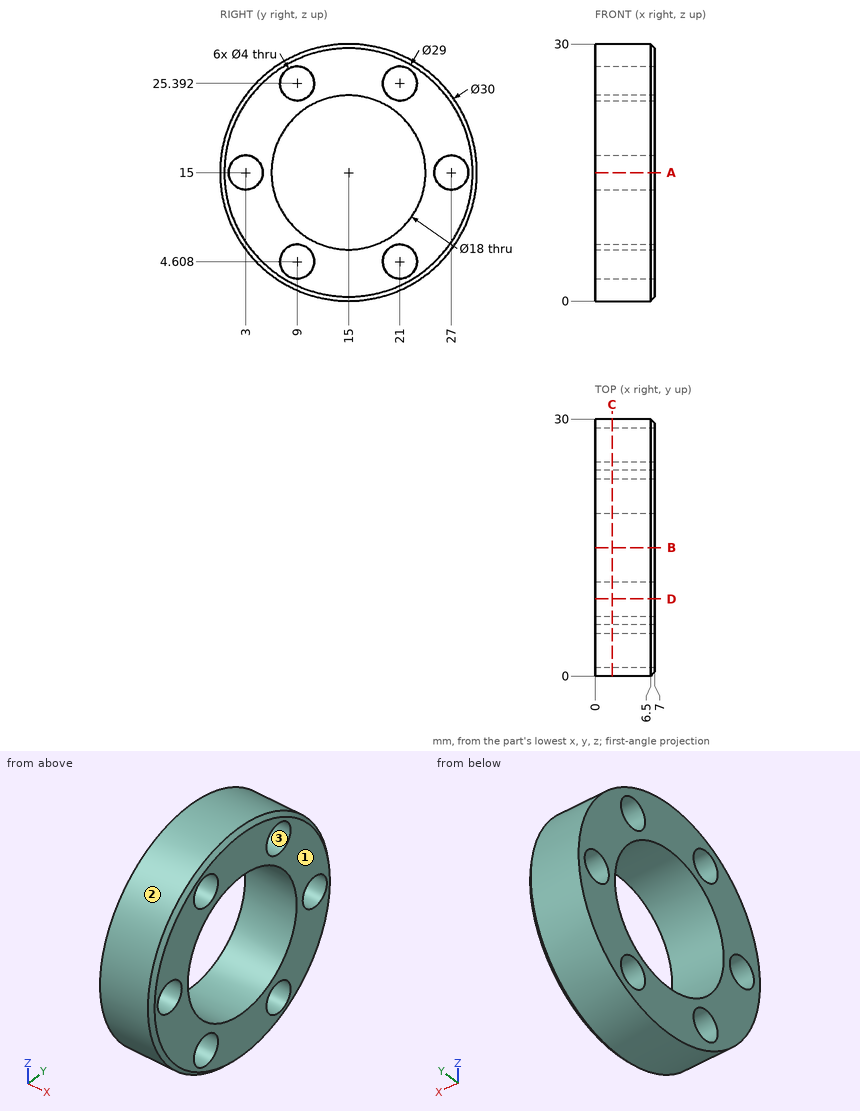
Check sheet for the drawn part. Datum: minimum x, y, z corner. Units: mm. Round coordinates to 2 decimals unless told otherwise and drop trailing zeros. Write each loop counter-clockwise with the first axis right and the second up, starting at its lowest first coordinate (ties: lowest second). Pieces come first, ordered by that corner, then holes. Notation, with made-up numbers: (73.25, -12) - (105.25, -12) arc R21 cw to (105.25, 8) - close; hole circle Ø1 at (59, 68.5). An arc over 180 degrees is marked (long way). Write each question's results on one line, items separated by ' | '.
(1) Depth check by flat-ended pin: pin 1 Ø2 at (x, z) = (4, 18.5) entering from -Y; pin 2 Ø1 at (x, z) = (1.5, 21) entering from -Y (1 decimal); pin 3 Ø2 at (x, z) = (6, 10.5) entering from +Y. Enter the tip coordinate at first touch or a pass-through.
Computed:
pin 1: stops at y = 0.21 | pin 2: stops at y = 1 | pin 3: stops at y = 29.59
(2) Thickness scan on probe 1 along Y at (x, z) = (3.5, 15); probe 2 along Z at (x, y) = (1, 22.5) (1 decimal); probe 3 along Y at (x, z) = (4.75, 5.25) (1 decimal). Record the ranges inside material, lowest first. Write a range as from..to.
Computed:
probe 1: y = 0..1, 5..6, 24..25, 29..30 | probe 2: z = 2..3.3, 5.9..10, 20..24.1, 26.7..28 | probe 3: y = 3.6..7.1, 10.9..19.1, 22.9..26.4
(3) Sectioned sample at D-D, the plane y = 9. Count the separate pieces of the cut face and the enclosed holes in it.
Computed:
separate pieces: 4 | enclosed holes: 0
(4) Draft check along Y on the marked faces 1, 2 and 3. Enter one of: pulls with the +Y half, pulls with the -Y half, needs draft (parallel to the pull), parting line crosses it, or undercut.
Computed:
face 1: needs draft | face 2: parting line crosses it | face 3: undercut
(5) Sectioned sample at A-A, the plane z = 15. Enter the section's corners in (x, y).
Computed:
outline: (0, 0) - (6.5, 0) - (7, 0.5) - (7, 1) - (0, 1) - close; (0, 5) - (7, 5) - (7, 6) - (0, 6) - close; (0, 24) - (7, 24) - (7, 25) - (0, 25) - close; (0, 29) - (7, 29) - (7, 29.5) - (6.5, 30) - (0, 30) - close
(6) Sectioned sample at C-C, the plane x = 2. Enter the section's corners in (y, z).
Computed:
outline: circle Ø30 at (15, 15); hole circle Ø4 at (3, 15); hole circle Ø18 at (15, 15); hole circle Ø4 at (9, 4.61); hole circle Ø4 at (9, 25.39); hole circle Ø4 at (21, 4.61); hole circle Ø4 at (21, 25.39); hole circle Ø4 at (27, 15)
(7) Sectioned sample at B-B, the plane y = 15. Enter the section's corners in (x, z).
Computed:
outline: (0, 0) - (6.5, 0) - (7, 0.5) - (7, 6) - (0, 6) - close; (0, 24) - (7, 24) - (7, 29.5) - (6.5, 30) - (0, 30) - close
